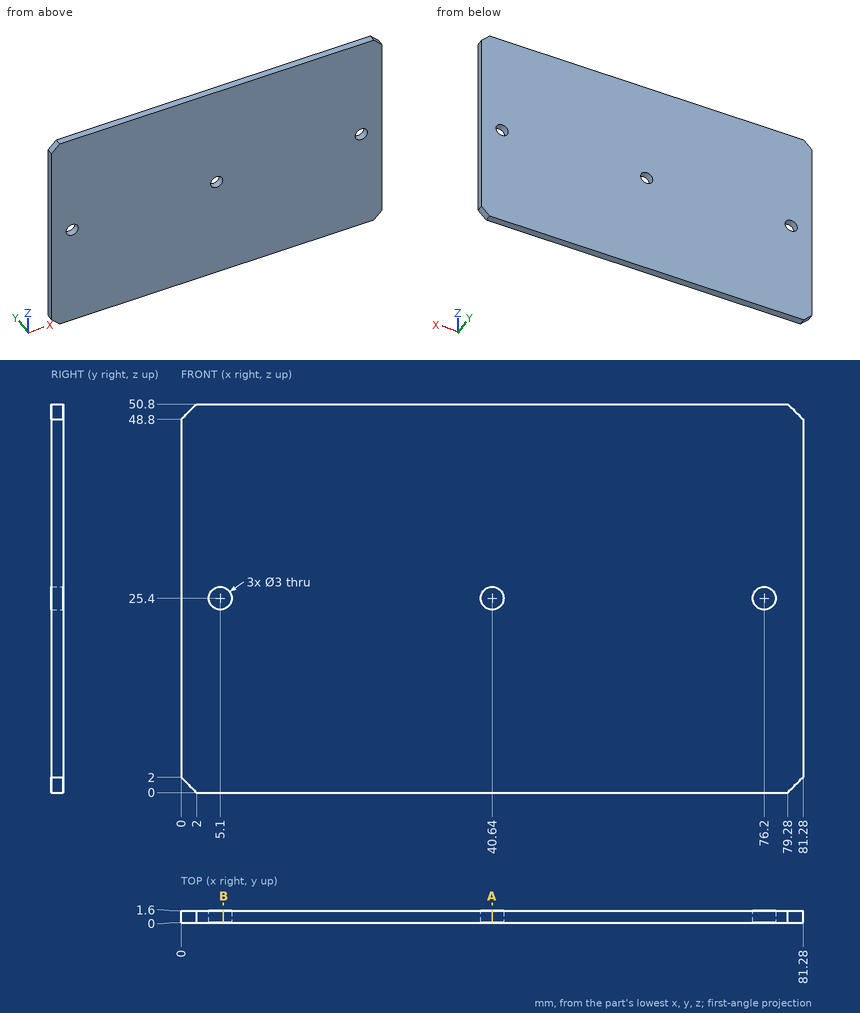
Part print with two shaded views. Sizes in mm from the minimum x, y, z corner. Coordinates: 2 decimals unless noted, no trailing zeros. Write each loop counter-clockwise with the first axis right and the second up, starting at its lowest first coordinate (ties: lowest second). Pieces come first, ordered by that corner, then holes. Notation, with made-up numbers: (-3, 65.5) - (33, 65.5) arc R25 cw to (33, 85.5) - close; hole circle Ø6 at (5, 19). An arc over 180 degrees is marked (long way). One line per item, written item: value. Start each with the question number.
1. Slice it at B-B (x = 5.5). Write the cut outline in (y, z).
2. Probe line 1 (X direction, y = 0.3, z = 25.4); line 2 (Z direction, x = 5.1, y = 0.4); line 3 (Z direction, x = 4.5, y = 1.55) (1 decimal). List the from-to ranges inside material, lowest first. Write a range as from..to.
3. Slice it at A-A (x = 40.64). Write the cut outline in (y, z).
Answers below:
1. outline: (0, 0) - (1.6, 0) - (1.6, 23.95) - (0, 23.95) - close; (0, 26.85) - (1.6, 26.85) - (1.6, 50.8) - (0, 50.8) - close
2. line 1: x = 0..3.6, 6.6..39.14, 42.14..74.7, 77.7..81.28
2. line 2: z = 0..23.9, 26.9..50.8
2. line 3: z = 0..24, 26.8..50.8
3. outline: (0, 0) - (1.6, 0) - (1.6, 23.9) - (0, 23.9) - close; (0, 26.9) - (1.6, 26.9) - (1.6, 50.8) - (0, 50.8) - close
